Can you work these out from the drawing? Everything is in mm from the part's minimum corner. A direction names the side the tool comes from. Round coordinates to 2 decimals unless told otherwise and drop trailing zeros. Write each loop counter-clockwise with the first axis right and the second up, starting at its lowest first coordinate (ties: lowest second). Pieces come first, ordered by that corner, then holes. Notation, with made-up numbers: (-24, 62.25) -> (31, 62.25) arc R18 cw to (31, 72.25) -> close; hole circle Ø8 at (17, 57). An arc over 180 degrees is marked (long way). Write item = value, one per line. Start each with the question number.
1) Imagine slicing it at D-D, the plane z = 35.25. Please give me the cut outline in (x, y).
2) If I drill on line 1 (Z direction, x = 20, y = 2.25); line 2 (X direction, y = 7.5, z = 35.25); line 3 (X direction, y = 21.75, z = 53.5), over which ranges is the centre line in solid material (lowest first)?
3) Imagine slicing it at A-A, the plane z = 72. Please give me the cut outline in (x, y).
4) Imagine slicing it at C-C, the plane y = 4. Please give me the cut outline in (x, z).
5) Imagine slicing it at B-B, the plane x = 20. Please give me the cut outline in (y, z).
6) I'm going to push flat-ended pins straight in: pin 1 (5.5 mm diameter, centred on x = 20, z = 12, fed in from -Y); pin 2 (1 mm diameter, centred on x = 12, y = 20, fed in from -Z); pin 3 (5 mm diameter, centred on x = 23, z = 72, fed in from -Y); pin 4 (3 mm diameter, centred on y = 8.5, z = 28.5, fed in from +X). Where does each tip first touch, or does it pass through?
7) For the marked faces 1, 2, 3, 4 and 5, which set-ups out of +Z, -Z, +X, -X, +Y, -Y let a thin tool reach every point of the face, with its end or its side?
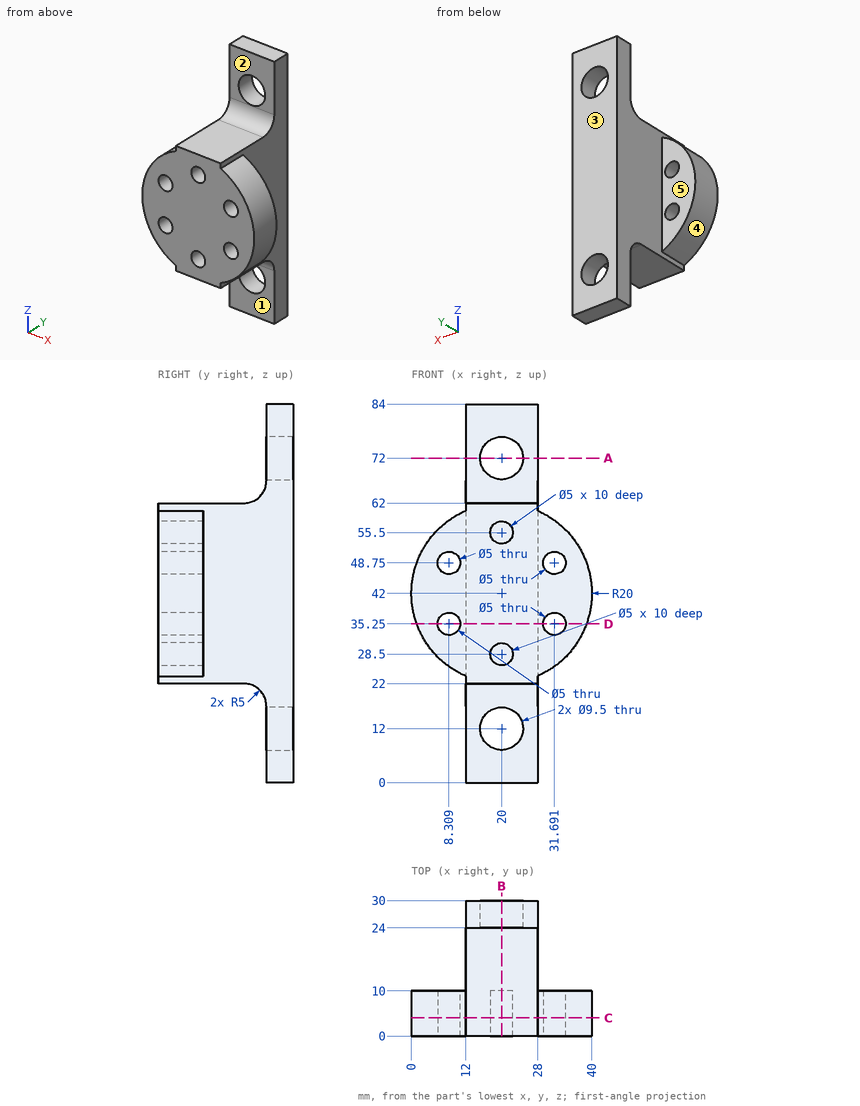
Reported:
q1.outline = (1.17, 0) -> (5.81, 0) -> (5.81, 10) -> (1.17, 10) -> close; (10.81, 0) -> (29.19, 0) -> (29.19, 10) -> (28, 10) -> (28, 30) -> (12, 30) -> (12, 10) -> (10.81, 10) -> close; (34.19, 0) -> (38.83, 0) -> (38.83, 10) -> (34.19, 10) -> close
q2.line_1 = 22 to 26, 31 to 53, 58 to 62
q2.line_2 = 1.17 to 5.81, 10.81 to 29.19, 34.19 to 38.83
q2.line_3 = 12 to 28
q3.outline = (12, 24) -> (15.25, 24) -> (15.25, 30) -> (12, 30) -> close; (24.75, 24) -> (28, 24) -> (28, 30) -> (24.75, 30) -> close
q4.outline = (12, 22) -> (28, 22) -> (28, 23.67) arc R20 ccw to (28, 60.33) -> (28, 62) -> (12, 62) -> (12, 60.33) arc R20 ccw to (12, 23.67) -> close; hole circle Ø5 at (8.31, 35.25); hole circle Ø5 at (8.31, 48.75); hole circle Ø5 at (20, 28.5); hole circle Ø5 at (20, 55.5); hole circle Ø5 at (31.69, 35.25); hole circle Ø5 at (31.69, 48.75)
q5.outline = (0, 22) -> (19, 22) arc R5 cw to (24, 17) -> (24, 16.75) -> (30, 16.75) -> (30, 67.25) -> (24, 67.25) -> (24, 67) arc R5 cw to (19, 62) -> (0, 62) -> (0, 58) -> (10, 58) -> (10, 53) -> (0, 53) -> (0, 31) -> (10, 31) -> (10, 26) -> (0, 26) -> close; (24, 0) -> (30, 0) -> (30, 7.25) -> (24, 7.25) -> close; (24, 76.75) -> (30, 76.75) -> (30, 84) -> (24, 84) -> close
q6.pin_1 = through
q6.pin_2 = 21.77
q6.pin_3 = 24
q6.pin_4 = 36
q7.face_1 = -Z, +X, -X, -Y
q7.face_2 = +Z, +X, -X, -Y
q7.face_3 = +Z, -Z, +X, -X, +Y
q7.face_4 = -X, +Y, -Y
q7.face_5 = +Z, -Z, -X, +Y
